The model under review builds one solid part; all positions refer to its coordinate system, in mm. Round coordinates to 2 decimals unless told otherwise and drop trailing zeros. Write each loop counter-clockwise with the first axis right and the second up, starting at its lowest first coordinate (ties: lowest second). Pieces come first, ordered by that corner, then holes. Notation, with made-up numbers: (-39.75, 44) -> (-29.75, 44) arc R27 cw to (-29.75, 66) -> close; hole circle Ø5 at (17.5, -13). An arc over 180 degrees is marked (long way). Answer as a JSON object with one key per item and string values. Group by question number.
1) Insertion check: pin 1 Ø5 at (x, z) = (12, -4) entering from +Y; pin 2 Ø3 at (x, y) = (83.5, 4) entering from -Z. Each pin has a flat end and moves straight along its axis. Give the tip position at first contact, or say it passes through.
2) We need section A-A, the plane z = -4. Write out the cut boundary in (x, y), then the cut area to 3 significant figures.
3) We need section B-B, the plane x = 12. Write out the cut boundary in (y, z), then the cut area to 4 significant figures.
4) We need section D-D, the plane x = 25. Write out the cut boundary in (y, z), then the cut area to 4 significant figures.
5) We need section C-C, the plane y = 3.65. Write out the cut boundary in (x, z), then the cut area to 3 significant figures.
6) To check wall thickness, follow probe 1 along X at (y, z) = (1.1, -4); probe 2 along X at (y, z) = (4.15, -4); probe 3 along Z at (x, y) = (12, 1.35). State the ranges of each line that lie inside material, in increasing order. Write a range as [from, to].
Autodesk Inventor part; units mm, degrees
ref_plane "YZ Plane" through (0, 0, 0) normal (1, 0, 0) x (0, 1, 0)
ref_plane "XZ Plane" through (0, 0, 0) normal (0, 1, 0) x (-1, 0, 0)
ref_plane "XY Plane" through (0, 0, 0) normal (0, 0, 1) x (1, 0, 0)
sketch "Sketch1" plane through (0, 0, 0) normal (1, 0, 0) x (0, 1, 0)
  line L0 (0, 0) -> (5, 0)
  line L1 (5, 0) -> (5, -10)
  line L2 (5, -10) -> (2.5, -7.5)
  line L3 (2.5, -7.5) -> (0, -10)
  line L4 (0, 0) -> (0, -10)
  line L5 (2.5, -7.5) -> (2.5, -12.5) construction
  circle A0 centre (2.5, -10.3284) radius 2 construction
  line L6 (2.5, -10.3284) -> (1.25, -10.3284) construction
  line L7 (5, -10.6569) -> (2.5, -13.1569) construction
  line L8 (2.5, -13.1569) -> (0, -10.6569) construction
  dimension "d0" = 5
  dimension "d3" = 10
  dimension "d4" = 4
  dimension "d33" = 0.6569
  dimension "d34" = 5.6569
  dimension "d35" = 2.8284
extrude "Extrusion1" add sketch "Sketch1" along normal blind 100
sketch "Sketch2" plane through (0, 5, 0) normal (0, 1, 0) x (1, 0, 0)
  line L0 (0, 10) -> (0, 0) construction
  line L1 (0, 0) -> (100, 0) construction
  line L2 (0, 10) -> (100, 10) construction
  line L3 (12, 0) -> (12, 10) construction
  line L4 (50, 0) -> (50, 15) construction
  circle A0 centre (12, 4) radius 2
  circle A1 centre (88, 4) radius 2
  point P0 (0, 5)
  dimension "d8" = 10
  dimension "d10" = 12
  dimension "d12" = 15
  dimension "d13" = 50
  dimension "d14" = 4
  dimension "d15" = 4
hole "Hole1" at (12, 5, -4) direction (0, -1, 0) diameter 4 end through all counterbore diameter 6 counterbore depth 3
hole "Hole2" at (88, 5, -4) direction (0, -1, 0) diameter 4 end through all counterbore diameter 6 counterbore depth 3
sketch "Sketch3" plane through (100, 0, 0) normal (1, 0, 0) x (0, 0, -1)
  line L0 (0, 5) -> (0, 0)
  line L1 (0, 2.5) -> (3, 2.5) construction
  circle A0 centre (3, 2.5) radius 1.6
  dimension "d36" = 3
  dimension "d37" = 3.2
hole "Hole3" [suppressed]
chamfer "Chamfer2" [suppressed]
sketch "Sketch4" plane through (0, 0, 0) normal (-1, 0, 0) x (0, 0, 1)
  line L0 (0, 5) -> (0, 0)
  circle A0 centre (-3, 2.5) radius 1.7294
  line L1 (0, 2.5) -> (-3, 2.5)
  circle A1 centre (-3, 2.5) radius 1.6
  line L2 (0, 5) -> (0, 0)
  dimension "d48" = 3.2
  dimension "d59" = 3
hole "Hole4" [suppressed]
chamfer "Chamfer3" [suppressed]
properties part number "K-tor-kulek" material "Steel, High Strength, Low Alloy"
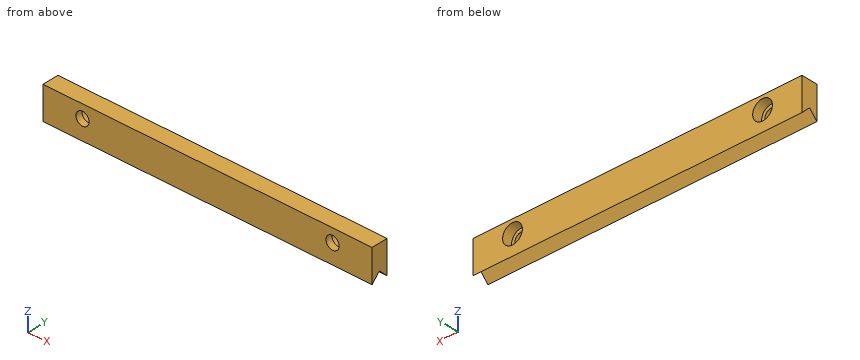
Here are the results:
{
 "1": {"pin 1": "stops at y = 2", "pin 2": "stops at z = -10"},
 "2": {"outline": "(0, 0) -> (10, 0) -> (10, 2) -> (9, 2) -> (9, 5) -> (0, 5) -> close; (14, 0) -> (86, 0) -> (86, 2) -> (85, 2) -> (85, 5) -> (15, 5) -> (15, 2) -> (14, 2) -> close; (90, 0) -> (100, 0) -> (100, 5) -> (91, 5) -> (91, 2) -> (90, 2) -> close", "area": "448 mm^2"},
 "3": {"outline": "(0, -10) -> (2.5, -7.5) -> (5, -10) -> (5, -7) -> (2, -7) -> (2, -6) -> (0, -6) -> close; (0, -2) -> (2, -2) -> (2, -1) -> (5, -1) -> (5, 0) -> (0, 0) -> close", "area": "17.75 mm^2"},
 "4": {"outline": "(0, -10) -> (2.5, -7.5) -> (5, -10) -> (5, 0) -> (0, 0) -> close", "area": "43.75 mm^2"},
 "5": {"outline": "(0, -8.65) -> (100, -8.65) -> (100, 0) -> (0, 0) -> close; hole circle Ø6 at (12, -4); hole circle Ø6 at (88, -4)", "area": "808 mm^2"},
 "6": {"probe 1": "x = [0, 10], [14, 86], [90, 100]", "probe 2": "x = [0, 9], [15, 85], [91, 100]", "probe 3": "z = [-8.65, -6], [-2, 0]"}
}
